Could you check a few things on this model? Use its own coordinates, in mm. A direction names the side the tool comes from. Round coordinates to 2 decimals unless told otherwise and drop trailing zeros. Loops run counter-clockwise (first coordinate to the right, second up) from the corner with the lowest first, then second, coordinate; pieces in that order, holes last. Notation, with made-up numbers: (-16, -34) -> (-1, -34) arc R23 cw to (-1, -22) -> close; hole circle Ø4 at (83, 35). An arc over 180 degrees is marked (long way). One line per item, written item: value.
```python
from build123d import *

# Parameters (mm, degrees)
F0_R     = 3.81
F1_DEPTH = 6.35
F2_W     = 6.35
F2_H     = 9.5123
F3_DEPTH = 15.875
F4_R     = 1.27
F6_DEPTH = 6.351


with BuildPart() as f1:
    # F0 (on Top) → F1 (new body)
    with BuildSketch(Plane.XY):
        with BuildLine():
            ThreePointArc((-6.1483610621, -4.7625), (-4.5608610621, -4.9641389379), (-3.0741805311, -5.55625))
            ThreePointArc((-3.0741805311, -5.55625), (6.3499966259, 0.0065460587), (-3.0856295938, 5.5499))
            ThreePointArc((-3.0856295938, 5.5499), (-4.577421837, 4.9530787195), (-6.1712591876, 4.7498))
            Line((-6.1712591876, 4.7498), (-31.75, 4.7498))
            Line((-31.75, 4.7498), (-31.75, -4.7625))
            Line((-31.75, -4.7625), (-6.1483610621, -4.7625))
        make_face()
        Circle(F0_R, mode=Mode.SUBTRACT)
    extrude(amount=F1_DEPTH)

    # F2 (on face) → F3 (join)
    with BuildSketch(Plane.XY.offset(6.35)):
        with Locations((-28.575, -0.00635)):
            Rectangle(F2_W, F2_H)
        with Locations((-14.605, -0.00635)):
            Rectangle(F2_W, F2_H)
    extrude(amount=F3_DEPTH)

    # F4
    f4_edges = [f1.edges().sort_by_distance(p)[0] for p in [
        (-18.949181, -4.7625, 0),
        (-8.789181, -4.7625, 6.35),
        (-11.43, -0.00635, 6.35),
        (-11.43, -0.00635, 22.225),
        (-31.75, -4.7625, 11.1125),
        (-31.75, -0.00635, 0),
        (-31.75, 4.7498, 11.1125),
        (-28.575, -4.7625, 22.225),
        (-31.75, -0.00635, 22.225),
        (-28.575, 4.7498, 22.225),
        (-14.605, -4.7625, 22.225),
        (-14.605, 4.7498, 22.225),
        (-4.560861, -4.964139, 0),
        (-4.560861, -4.964139, 6.35),
        (-4.577422, 4.953079, 6.35),
        (-4.577422, 4.953079, 0),
        (-11.43, 4.7498, 14.2875),
        (-18.96063, 4.7498, 0),
        (-11.43, -4.7625, 14.2875),
    ]]
    fillet(f4_edges, radius=F4_R)

    # F5 (on Right) → F6 (cut, through all)
    with BuildSketch(Plane.YZ):
        Polygon((-4.3603489199, -4.6240965693), (-1.9896510801, -5.5359034307), (4.3603489199, 10.9740965693), (1.9896510801, 11.8859034307), align=None)
    extrude(amount=F6_DEPTH, mode=Mode.SUBTRACT)


solid = f1.part
```
Item 1: If we section it at C-C on x = -24: List the corners of the cut face in (y, z) for me.
Output:
outline: (-4.76, 1.27) arc R1.27 ccw to (-3.49, 0) -> (3.48, 0) arc R1.27 ccw to (4.75, 1.27) -> (4.75, 6.35) -> (-4.76, 6.35) -> close
Item 2: Will these pins go through, and if not, where does the flat tip stop? pin 1 Ø8 at (x, z) = (-15, 8.5) entering from -Y; pin 2 Ø3 at (x, y) = (-3, 3.5) entering from +Z; pin 3 Ø12 at (x, z) = (-10, 15) entering from +Y.
Output:
pin 1: stops at y = -4.76
pin 2: stops at z = 6.35
pin 3: stops at y = 4.75
Item 3: If we section it at A-A on z = 8.5: List the corners of the cut face in (x, y) for me, plus the area to 3 significant figures.
Output:
outline: (-31.75, -3.49) arc R1.27 ccw to (-30.48, -4.76) -> (-25.4, -4.76) -> (-25.4, 4.75) -> (-30.48, 4.75) arc R1.27 ccw to (-31.75, 3.48) -> close; (-17.78, -4.76) -> (-12.7, -4.76) arc R1.27 ccw to (-11.43, -3.49) -> (-11.43, 3.48) arc R1.27 ccw to (-12.7, 4.75) -> (-17.78, 4.75) -> close
area: 119 mm²
Item 4: If we mould it in two halves opening along X, with no side actions, what happens to faces 1 (the face through (-11.792, 4.368, 14.381)), 2 (the face through (-17.78, 0, 14)), 3 (the face through (4.928, -1.344, 3.219)), 4 (the face through (-31.388, -0.055, 0.382))? For each: released by +X, released by -X, zero draft, split by the parting line, or undercut.
Output:
face 1: released by +X
face 2: undercut
face 3: zero draft
face 4: released by -X
Item 5: If we section it at B-B on x = -14.5: List the corners of the cut face in (y, z) for me (1 decimal).
Output:
outline: (-4.8, 1.3) arc R1.3 ccw to (-3.5, 0) -> (3.5, 0) arc R1.3 ccw to (4.7, 1.3) -> (4.7, 21) arc R1.3 ccw to (3.5, 22.2) -> (-3.5, 22.2) arc R1.3 ccw to (-4.8, 21) -> close
Item 6: For faces 5 (the face through (-11.81, -4.4, 14.38)), 6 (the face through (-25.4, 0, 14)), 7 (the face through (-16, -4.762, 9)), which set-ups out of +Z, -Z, +X, -X, +Y, -Y let a thin tool reach every point of the face, with its end or its side?
Output:
face 5: +Z, +X, -Y
face 6: +Z, +Y, -Y
face 7: +Z, -Z, -X, -Y
Item 7: I need wall thicknesses on line 1 (Y direction, x = 0, z = 3); line 2 (X direction, y = 1, z = 19.25); line 3 (X direction, y = 0, z = 4). Which ranges of each line are inside material? Lowest first, please. Write a range as from..to.
Output:
line 1: y = -6.35..-3.81, 3.81..6.35
line 2: x = -31.75..-25.4, -17.78..-11.43
line 3: x = -31.75..-3.81
